```python
from build123d import *

# Parameters (mm, degrees)
BOSS_EXTRUDE1_DEPTH = 20
SKETCH2_R           = 2.75
CUT_EXTRUDE1_DEPTH  = 5
FILLET1_R           = 1
SKETCH7_W           = 42
SKETCH7_H           = 12
CUT_EXTRUDE3_DEPTH  = 5
SKETCH9_R           = 2.25
CUT_EXTRUDE5_DEPTH  = 56.479726027
FILLET3_R           = 15
FILLET4_R           = 3
FILLET5_R           = 3


# Some blends are built 0.0001 mm under size
with BuildPart() as part:
    # Sketch1 → Boss-Extrude1 (new body)
    with BuildSketch(Plane(origin=(0, 0, 0), x_dir=(1, 0, 0), z_dir=(0, 1, 0))):
        Polygon((21, -30), (-21, -30), (-21, -6), (-20, -6), (-20, 0), (-33, 0), (-33, -42), (33, -42), (33, 0), (20, 0), (20, -6), (21, -6), align=None)
    extrude(amount=BOSS_EXTRUDE1_DEPTH)

    # Sketch2 → Cut-Extrude1 (cut)
    with BuildSketch(Plane(origin=(0, 0, 0), x_dir=(-1, 0, 0), z_dir=(0, 0, -1))):
        with Locations((-24.25, 14.79)):
            Circle(SKETCH2_R)
        with Locations((-24.25, 4.79)):
            Circle(SKETCH2_R)
    cut_extrude1 = extrude(amount=-CUT_EXTRUDE1_DEPTH, mode=Mode.SUBTRACT)

    # Mirror1: Cut-Extrude1 across plane
    add(cut_extrude1.mirror(Plane(origin=(0, 0, 0), x_dir=(0, 0, 1), z_dir=(1, 0, 0))), mode=Mode.SUBTRACT)

    # Fillet1
    fillet1_edges = [part.edges().sort_by_distance(p)[0] for p in [
        (-20, 10, 0),
        (20, 10, 0),
        (20, 10, 6),
        (-20, 10, 6),
    ]]
    fillet(fillet1_edges, radius=FILLET1_R - 0.0001)  # a hair under: the kernel refuses the full size

    # Sketch7 → Cut-Extrude3 (cut)
    with BuildSketch(Plane.XZ):
        Polygon((-33, 6), (-21, 6), (-21, 30), (-21, 42), (-33, 42), align=None)
        with Locations((0, 36)):
            Rectangle(SKETCH7_W, SKETCH7_H)
        Polygon((21, 42), (21, 30), (21, 6), (33, 6), (33, 42), align=None)
    cut_extrude3 = extrude(amount=-CUT_EXTRUDE3_DEPTH, mode=Mode.SUBTRACT)

    # Mirror2: Cut-Extrude3 across plane
    add(cut_extrude3.mirror(Plane.ZX.offset(10)), mode=Mode.SUBTRACT)

    # Sketch9 → Cut-Extrude5 (cut, through all)
    with BuildSketch(Plane.XZ.offset(-5)):
        with Locations(Location((-27, 17.5, 0), (0, 0, 270))):
            Circle(SKETCH9_R)
        with Locations(Location((27, 17.5, 0), (0, 0, 270))):
            Circle(SKETCH9_R)
        with Locations(Location((0, 36, 0), (0, 0, 270))):
            Circle(SKETCH9_R)
    extrude(amount=-CUT_EXTRUDE5_DEPTH, mode=Mode.SUBTRACT)

    # Fillet3
    fillet3_edges = [part.edges().sort_by_distance(p)[0] for p in [
        (-33, 10, 42),
        (33, 10, 42),
    ]]
    fillet(fillet3_edges, radius=FILLET3_R)

    # Fillet4
    fillet4_edges = [part.edges().sort_by_distance(p)[0] for p in [
        (-21, 10, 30),
        (21, 10, 30),
    ]]
    fillet(fillet4_edges, radius=FILLET4_R)

    # Fillet5
    # the kernel refuses this fillet: 3 mm, written as the material it takes off along each edge
    with BuildSketch(Plane(origin=(-33, 27.5, 6), x_dir=(1, 0, 0), z_dir=(0, -1, 0)), Plane(origin=(33, -7.5, 6), x_dir=(-1, 0, 0), z_dir=(0, 1, 0))) as fillet5_piece_1:
        with BuildLine():
            CenterArc((FILLET5_R, -FILLET5_R), FILLET5_R, 90, 90)
            Line((0, -FILLET5_R), (0, 0))
            Line((0, 0), (FILLET5_R, 0))
        make_face()
    extrude(amount=12.5, mode=Mode.SUBTRACT)
    with BuildSketch(Plane(origin=(33, 27.5, 6), x_dir=(-1, 0, 0), z_dir=(0, -1, 0)), Plane(origin=(-33, -7.5, 6), x_dir=(1, 0, 0), z_dir=(0, 1, 0))) as fillet5_piece_2:
        with BuildLine():
            CenterArc((FILLET5_R, FILLET5_R), FILLET5_R, 180, 90)
            Line((0, FILLET5_R), (0, 0))
            Line((0, 0), (FILLET5_R, 0))
        make_face()
    extrude(amount=12.5, mode=Mode.SUBTRACT)
    with BuildSketch(Plane(origin=(-33, -7.5, 0), x_dir=(0, 0, 1), z_dir=(0, 1, 0))) as fillet5_piece_3:
        with BuildLine():
            CenterArc((FILLET5_R, FILLET5_R), FILLET5_R, 180, 90)
            Line((0, FILLET5_R), (0, 0))
            Line((0, 0), (FILLET5_R, 0))
        make_face()
    extrude(amount=35, mode=Mode.SUBTRACT)
    with BuildSketch(Plane(origin=(33, -7.5, 0), x_dir=(0, 0, 1), z_dir=(0, 1, 0))) as fillet5_piece_4:
        with BuildLine():
            CenterArc((FILLET5_R, -FILLET5_R), FILLET5_R, 90, 90)
            Line((0, -FILLET5_R), (0, 0))
            Line((0, 0), (FILLET5_R, 0))
        make_face()
    extrude(amount=35, mode=Mode.SUBTRACT)


solid = part.part
```
Model file for the job. Use its own axes, mm. A direction names the side the tool comes from. Coordinates: 2 decimals unless noted, no trailing zeros. Order: outer loops, then holes, each group sorted by start corner. A loop starts at its lowest first (then second) coordinate and runs counter-clockwise, first axis right, second up. Notation, with made-up numbers: (78, 40.25) - (115, 40.25) arc R35 cw to (115, 78.25) - close; hole circle Ø5 at (70.5, -12.5). An arc over 180 degrees is marked (long way). Return JSON: item names as keys, results as strings. Group by question number.
1) Saw through at D-D, the plane z = 17. Write the cut outline in (x, y).
2) Saw through at B-B, the plane z = 11. Write the cut outline in (x, y).
3) Tool access for faces 5 (the cylindrical face through (-32.796, 9.86, 1.912)), 6 (the flat face through (20, 10, 3)), 7 (the cylindrical face through (20.1, 10.07, 29.14)), 8 (the flat face through (-24, 5, 5)), 9 (the flat face through (25, 3, 6)): list every direction of +Z, -Z, +X, -X, +Y, -Y with a clear straight run to the whole face (end or side of a thin tool).
4) Saw through at C-C, the plane y = 9. Count the separate pieces of the cut face and the enclosed holes in it, plus the area to 3 significant figures.
5) Saw through at A-A, the plane x = 0. Write the cut outline in (y, z).
6) Mould opens along Y. For faces 1 (the cylindrical face through (26.997, 4.911, 2.465)), 2 (the cylindrical face through (-26.997, 4.911, 2.465)), 3 (the flat face through (0, 15, 31)), 4 (the flat face through (26, 10, 0)) say: released by +Y, released by -Y, zero draft, split by the parting line, or undercut.
7) Probe line 1 (X direction, y = 9.5, z = 17.5); line 2 (Y direction, x = -24.25, z = 3.6); line 3 (X direction, y = 10.75, z = 16.5). List the from-to ranges inside material, lowest first. Write a range as from..to.
8) Flat gauge pins, fed straight in: P1, Ø10, axis at x = 27.5, y = 7, coming from the +Z side; P2, Ø1.5, axis at y = 4, z = 5.5, coming from the -X side; P3, Ø10, axis at x = -27, y = 10.5, coming from the +Z side. Where does each tip first touch, or does it go through?
Values found:
{
 "1": {"outline": "(-33, 5) - (-29.19, 5) - (-29.19, 15) - (-33, 15) - close; (-24.81, 5) - (-21, 5) - (-21, 15) - (-24.81, 15) - close; (21, 5) - (24.81, 5) - (24.81, 15) - (21, 15) - close; (29.19, 5) - (33, 5) - (33, 15) - (29.19, 15) - close"},
 "2": {"outline": "(-33, 5) - (-21, 5) - (-21, 15) - (-33, 15) - close; (21, 5) - (33, 5) - (33, 15) - (21, 15) - close"},
 "3": {"face 5": "-X", "face 6": "-Z, +Y, -Y", "face 7": "+Y, -Y", "face 8": "-Z", "face 9": "+Z, +X, -X"},
 "4": {"separate pieces": "1", "enclosed holes": "3", "area": "1,380 mm²"},
 "5": {"outline": "(5, 30) - (15, 30) - (15, 33.75) - (5, 33.75) - close; (5, 38.25) - (15, 38.25) - (15, 42) - (5, 42) - close"},
 "6": {"face 1": "undercut", "face 2": "undercut", "face 3": "released by +Y", "face 4": "zero draft"},
 "7": {"line 1": "x = -33..-29.25, -24.75..-21, 21..24.75, 29.25..33", "line 2": "y = 0..2.04, 7.54..12.04, 17.54..20", "line 3": "x = -33..-29.02, -24.98..-21, 21..24.98, 29.02..33"},
 "8": {"P1": "stops at z = 41.31", "P2": "stops at x = -32.44", "P3": "stops at z = 41.46"}
}
